```python
from build123d import *

# Parameters (mm, degrees)
SKETCH1_W           = 25
SKETCH1_H           = 68.1
BOSS_EXTRUDE1_DEPTH = 31.05
CUT_EXTRUDE1_REACH  = 54.426
SKETCH2_W           = 15
SKETCH2_H           = 26.05
SKETCH3_W           = 17
SKETCH3_H           = 21.05
CUT_EXTRUDE2_DEPTH  = 25
SKETCH7_W           = 25
SKETCH7_H           = 38.1
BOSS_EXTRUDE2_DEPTH = 5
SKETCH11_W          = 25
SKETCH11_H          = 15
CUT_EXTRUDE3_DEPTH  = 5
FILLET1_R           = 3.175
FILLET2_R           = 0.5
FILLET3_R           = 3.175


with BuildPart() as part:
    # Sketch1 → Boss-Extrude1 (new body)
    with BuildSketch(Plane(origin=(0, 0, 0), x_dir=(1, 0, 0), z_dir=(0, 1, 0))):
        Rectangle(SKETCH1_W, SKETCH1_H)
    extrude(amount=-BOSS_EXTRUDE1_DEPTH)

    # Sketch2 → Cut-Extrude1 (cut, up to next)
    with BuildSketch(Plane(origin=(12.5, 0, 0), x_dir=(0, 0, -1), z_dir=(1, 0, 0)), mode=Mode.PRIVATE) as cut_extrude1_sk1:
        with Locations((-26.55, -18.025)):
            Rectangle(SKETCH2_W, SKETCH2_H)
    cut_extrude1_tool1 = extrude(cut_extrude1_sk1.sketch, amount=-CUT_EXTRUDE1_REACH, mode=Mode.PRIVATE) & part.part
    # Sketch2 → Cut-Extrude1 (cut, up to next)
    with BuildSketch(Plane(origin=(12.5, 0, 0), x_dir=(0, 0, -1), z_dir=(1, 0, 0)), mode=Mode.PRIVATE) as cut_extrude1_sk2:
        with Locations((26.55, -18.025)):
            Rectangle(SKETCH2_W, SKETCH2_H)
    cut_extrude1_tool2 = extrude(cut_extrude1_sk2.sketch, amount=-CUT_EXTRUDE1_REACH, mode=Mode.PRIVATE) & part.part
    add(cut_extrude1_tool1.solids().sort_by_distance((12.5, -18.025, 26.55))[0], mode=Mode.SUBTRACT)
    add(cut_extrude1_tool2.solids().sort_by_distance((12.5, -18.025, -26.55))[0], mode=Mode.SUBTRACT)

    # Sketch3 → Cut-Extrude2 (cut, symmetric)
    with BuildSketch(Plane.XY):
        with Locations((-4, -15.525)):
            Rectangle(SKETCH3_W, SKETCH3_H)
    extrude(amount=CUT_EXTRUDE2_DEPTH, both=True, mode=Mode.SUBTRACT)

    # Sketch6 → Cut-Revolve2 (revolve, cut)
    with BuildSketch(Plane.XY, mode=Mode.PRIVATE) as cut_revolve2_sk:
        Polygon((-4, 0), (-4, -5), (-0.75, -5), (-0.75, -4), (1.5, -4), (1.5, 0), align=None)
    revolve(cut_revolve2_sk.sketch.rotate(Axis((-4, 0, 0), (0, -1, 0)), 180), axis=Axis((-4, 0, 0), (0, -1, 0)), mode=Mode.SUBTRACT)

    # Sketch7 → Boss-Extrude2 (add)
    with BuildSketch(Plane(origin=(0, 0, 0), x_dir=(1, 0, 0), z_dir=(0, 1, 0))):
        with Locations((25, 0)):
            Rectangle(SKETCH7_W, SKETCH7_H)
    extrude(amount=-BOSS_EXTRUDE2_DEPTH)

    # Sketch10 → Cut-Revolve3 (revolve, cut)
    with BuildSketch(Plane.XY, mode=Mode.PRIVATE) as cut_revolve3_sk:
        Polygon((25, 0), (19, 0), (22.75, -3.75), (22.75, -5), (25, -5), align=None)
    revolve(cut_revolve3_sk.sketch.rotate(Axis((25, -5, 0), (0, 1, 0)), 270), axis=Axis((25, -5, 0), (0, 1, 0)), mode=Mode.SUBTRACT)

    # Sketch11 → Cut-Extrude3 (cut)
    with BuildSketch(Plane(origin=(0, 0, 0), x_dir=(1, 0, 0), z_dir=(0, 1, 0))):
        with Locations((0, 26.55)):
            Rectangle(SKETCH11_W, SKETCH11_H)
        with Locations((0, -26.55)):
            Rectangle(SKETCH11_W, SKETCH11_H)
    extrude(amount=-CUT_EXTRUDE3_DEPTH, mode=Mode.SUBTRACT)

    # Fillet1
    fillet1_edges = [part.edges().sort_by_distance(p)[0] for p in [
        (12.5, -18.025, 19.05),
        (12.5, -18.025, -19.05),
    ]]
    fillet(fillet1_edges, radius=FILLET1_R)

    # Fillet2
    fillet2_edges = [part.edges().sort_by_distance(p)[0] for p in [
        (-4, -5, 19.05),
        (12.5, -31.05, 0),
        (11.57006403, -31.05, -18.12006403),
        (11.57006403, -31.05, 18.12006403),
        (-12.5, -31.05, 0),
        (-1.5875, -31.05, 19.05),
        (-1.5875, -31.05, -19.05),
        (-4, -26.05, 19.05),
        (-12.5, -26.05, 0),
        (-4, -26.05, -19.05),
        (12.5, 0, -19.05),
        (12.5, 0, 19.05),
        (37.5, 0, 0),
        (23.4125, -5, -19.05),
        (37.5, -5, 0),
        (23.4125, -5, 19.05),
        (-12.5, -5, 0),
        (-4, -5, -19.05),
        (-12.5, 0, 0),
    ]]
    fillet(fillet2_edges, radius=FILLET2_R)

    # Fillet3
    # the kernel refuses this fillet: 3.175 mm, written as the material it takes off along each edge
    with BuildSketch(Plane(origin=(-9.325, -31.05, -15.875), x_dir=(-1, 0, 0), z_dir=(0, 0, 1))) as fillet3_piece_1:
        with BuildLine():
            CenterArc((2.675, -0.5), 0.5, 0, 90)
            Line((3.175, -0.5), (3.175, 0))
            Line((3.175, 0), (2.675, 0))
        make_face()
    revolve(axis=Axis((-9.325, -31.05, -15.875), (0, -1, 0)), revolution_arc=90, mode=Mode.SUBTRACT)
    with BuildSketch(Plane(origin=(-9.325, -31.05, 15.875), x_dir=(0, 0, 1), z_dir=(1, 0, 0))) as fillet3_piece_2:
        with BuildLine():
            CenterArc((2.675, -0.5), 0.5, 0, 90)
            Line((3.175, -0.5), (3.175, 0))
            Line((3.175, 0), (2.675, 0))
        make_face()
    revolve(axis=Axis((-9.325, -31.05, 15.875), (0, -1, 0)), revolution_arc=90, mode=Mode.SUBTRACT)
    with BuildSketch(Plane(origin=(-9.325, -26.05, -15.875), x_dir=(0, 0, -1), z_dir=(1, 0, 0))) as fillet3_piece_3:
        with BuildLine():
            CenterArc((2.675, -0.5), 0.5, 0, 90)
            Line((3.175, -0.5), (3.175, 0))
            Line((3.175, 0), (2.675, 0))
        make_face()
    revolve(axis=Axis((-9.325, -26.05, -15.875), (0, 1, 0)), revolution_arc=90, mode=Mode.SUBTRACT)
    with BuildSketch(Plane(origin=(-9.325, -26.05, 15.875), x_dir=(-1, 0, 0), z_dir=(0, 0, -1))) as fillet3_piece_4:
        with BuildLine():
            CenterArc((2.675, -0.5), 0.5, 0, 90)
            Line((3.175, -0.5), (3.175, 0))
            Line((3.175, 0), (2.675, 0))
        make_face()
    revolve(axis=Axis((-9.325, -26.05, 15.875), (0, 1, 0)), revolution_arc=90, mode=Mode.SUBTRACT)
    with BuildSketch(Plane(origin=(-9.325, 0, 15.875), x_dir=(-1, 0, 0), z_dir=(0, 0, -1))) as fillet3_piece_5:
        with BuildLine():
            CenterArc((2.675, -0.5), 0.5, 0, 90)
            Line((3.175, -0.5), (3.175, 0))
            Line((3.175, 0), (2.675, 0))
        make_face()
    revolve(axis=Axis((-9.325, 0, 15.875), (0, 1, 0)), revolution_arc=90, mode=Mode.SUBTRACT)
    with BuildSketch(Plane(origin=(-9.325, 0, -15.875), x_dir=(0, 0, -1), z_dir=(1, 0, 0))) as fillet3_piece_6:
        with BuildLine():
            CenterArc((2.675, -0.5), 0.5, 0, 90)
            Line((3.175, -0.5), (3.175, 0))
            Line((3.175, 0), (2.675, 0))
        make_face()
    revolve(axis=Axis((-9.325, 0, -15.875), (0, 1, 0)), revolution_arc=90, mode=Mode.SUBTRACT)
    with BuildSketch(Plane(origin=(34.325, 0, 15.875), x_dir=(0, 0, 1), z_dir=(-1, 0, 0))) as fillet3_piece_7:
        with BuildLine():
            CenterArc((2.675, -0.5), 0.5, 0, 90)
            Line((3.175, -0.5), (3.175, 0))
            Line((3.175, 0), (2.675, 0))
        make_face()
    revolve(axis=Axis((34.325, 0, 15.875), (0, 1, 0)), revolution_arc=90, mode=Mode.SUBTRACT)
    with BuildSketch(Plane(origin=(34.325, 0, -15.875), x_dir=(1, 0, 0), z_dir=(0, 0, 1))) as fillet3_piece_8:
        with BuildLine():
            CenterArc((2.675, -0.5), 0.5, 0, 90)
            Line((3.175, -0.5), (3.175, 0))
            Line((3.175, 0), (2.675, 0))
        make_face()
    revolve(axis=Axis((34.325, 0, -15.875), (0, 1, 0)), revolution_arc=90, mode=Mode.SUBTRACT)
    with BuildSketch(Plane(origin=(-9.325, -5, 15.875), x_dir=(0, 0, 1), z_dir=(1, 0, 0))) as fillet3_piece_9:
        with BuildLine():
            CenterArc((2.675, -0.5), 0.5, 0, 90)
            Line((3.175, -0.5), (3.175, 0))
            Line((3.175, 0), (2.675, 0))
        make_face()
    revolve(axis=Axis((-9.325, -5, 15.875), (0, -1, 0)), revolution_arc=90, mode=Mode.SUBTRACT)
    with BuildSketch(Plane(origin=(-9.325, -5, -15.875), x_dir=(-1, 0, 0), z_dir=(0, 0, 1))) as fillet3_piece_10:
        with BuildLine():
            CenterArc((2.675, -0.5), 0.5, 0, 90)
            Line((3.175, -0.5), (3.175, 0))
            Line((3.175, 0), (2.675, 0))
        make_face()
    revolve(axis=Axis((-9.325, -5, -15.875), (0, -1, 0)), revolution_arc=90, mode=Mode.SUBTRACT)
    with BuildSketch(Plane(origin=(34.325, -5, -15.875), x_dir=(0, 0, -1), z_dir=(-1, 0, 0))) as fillet3_piece_11:
        with BuildLine():
            CenterArc((2.675, -0.5), 0.5, 0, 90)
            Line((3.175, -0.5), (3.175, 0))
            Line((3.175, 0), (2.675, 0))
        make_face()
    revolve(axis=Axis((34.325, -5, -15.875), (0, -1, 0)), revolution_arc=90, mode=Mode.SUBTRACT)
    with BuildSketch(Plane(origin=(34.325, -5, 15.875), x_dir=(1, 0, 0), z_dir=(0, 0, -1))) as fillet3_piece_12:
        with BuildLine():
            CenterArc((2.675, -0.5), 0.5, 0, 90)
            Line((3.175, -0.5), (3.175, 0))
            Line((3.175, 0), (2.675, 0))
        make_face()
    revolve(axis=Axis((34.325, -5, 15.875), (0, -1, 0)), revolution_arc=90, mode=Mode.SUBTRACT)
    with BuildSketch(Plane(origin=(37.5, 0, 19.05), x_dir=(0, 0, -1), z_dir=(0, -1, 0)), Plane(origin=(-12.5, -31.05, 19.05), x_dir=(0, 0, -1), z_dir=(0, 1, 0)), Plane(origin=(-12.5, -31.05, -19.05), x_dir=(1, 0, 0), z_dir=(0, 1, 0)), Plane(origin=(37.5, 0, -19.05), x_dir=(-1, 0, 0), z_dir=(0, -1, 0))) as fillet3_piece_13:
        with BuildLine():
            CenterArc((FILLET3_R, -FILLET3_R), FILLET3_R, 90, 90)
            Line((0, -FILLET3_R), (0, 0))
            Line((0, 0), (FILLET3_R, 0))
        make_face()
    extrude(amount=5, mode=Mode.SUBTRACT)
    with BuildSketch(Plane(origin=(-12.5, 0, 19.05), x_dir=(0, 0, -1), z_dir=(0, -1, 0)), Plane(origin=(-12.5, 0, -19.05), x_dir=(1, 0, 0), z_dir=(0, -1, 0))) as fillet3_piece_14:
        with BuildLine():
            CenterArc((FILLET3_R, FILLET3_R), FILLET3_R, 180, 90)
            Line((0, FILLET3_R), (0, 0))
            Line((0, 0), (FILLET3_R, 0))
        make_face()
    extrude(amount=5, mode=Mode.SUBTRACT)


solid = part.part
```
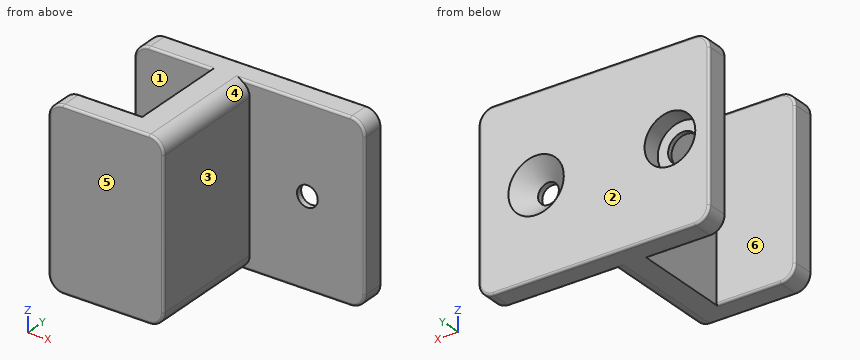
CAD build for the part. Positions are in the model's coordinates, mm. Face numbers are marked on the shaded views. A direction names the side the tool comes from. Round coordinates to 2 decimals unless told otherwise and drop trailing zeros. Order: outer loops, then holes, each group sorted by start corner. A loop starts at its lowest first (then second) coordinate and runs counter-clockwise, first axis right, second up.
Item 1: Saw through at B-B on z = 0. State how many separate pieces and enclosed holes the cut face has, then the cut area to 3 significant figures.
Item 2: Tool access for the marked faces 1, 2 and 3: list every direction of +Z, -Z, +X, -X, +Y, -Y with a clear straight run to the whole face (end or side of a thin tool).
Item 3: Saw through at C-C on x = -4. Write the cut outline in (y, z), then the cut area to 3 significant figures.
Item 4: Saw through at D-D on z = -14. Write the cut outline in (x, y).
Item 5: Saw through at A-A on x = 25. Write the cut outline in (y, z), then the cut area to 3 significant figures.
Item 6: Mould opens along Y. For the marked faces 4, 5 and 6 say: pulls with the +Y half, pulls with the -Y half, needs draft (parallel to the pull), parting line crosses it, or undercut.
Item 7: Probe line 1 along Y through (x, z) = (-3, -14); line 2 along X through (y, z) = (-1, -2); line 3 along Z through (x, y) = (-4, -4.6). List the from-to ranges inside material, lowest first.
Item 8: Pin check, flat tips, straight feed: pin 1 (8 mm diameter, centred on x = 23, z = 0, fed in from -Y); pin 2 (9 mm diameter, centred on x = -2, z = -1.5, fed in from +Y); pin 3 (1 mm diameter, centred on x = 12, y = -7, fed in from +Z); pin 4 (10.5 mm diameter, centred on x = -4, z = 0, fed in from +Y). Stop position of each tip, or through.
Reported:
1. separate pieces: 3
1. enclosed holes: 0
1. area: 456 mm2
2. face 1: +Z, -Z, -X
2. face 2: +Z, -Z, +X, -X, +Y
2. face 3: +Z, -Z, +X, -Y
3. outline: (-31.05, -18.55) arc R0.5 ccw to (-30.55, -19.05) - (-26.55, -19.05) arc R0.5 ccw to (-26.05, -18.55) - (-26.05, 18.55) arc R0.5 ccw to (-26.55, 19.05) - (-30.55, 19.05) arc R0.5 ccw to (-31.05, 18.55) - close; (-5, -18.55) arc R0.5 ccw to (-4.5, -19.05) - (-0.5, -19.05) arc R0.5 ccw to (0, -18.55) - (0, -5.5) - (-4, -5.5) - (-4, -3.25) - (-5, -3.25) - close; (-5, 3.25) - (-4, 3.25) - (-4, 5.5) - (0, 5.5) - (0, 18.55) arc R0.5 ccw to (-0.5, 19.05) - (-4.5, 19.05) arc R0.5 ccw to (-5, 18.55) - close
3. area: 330 mm2
4. outline: (-12.5, -30.55) arc R0.5 ccw to (-12, -31.05) - (12, -31.05) arc R0.5 ccw to (12.5, -30.55) - (12.5, -5) - (37, -5) arc R0.5 ccw to (37.5, -4.5) - (37.5, -0.5) arc R0.5 ccw to (37, 0) - (-12, 0) arc R0.5 ccw to (-12.5, -0.5) - (-12.5, -4.5) arc R0.5 ccw to (-12, -5) - (4.5, -5) - (4.5, -26.05) - (-12, -26.05) arc R0.5 ccw to (-12.5, -26.55) - close
5. outline: (-5, -18.55) arc R0.5 ccw to (-4.5, -19.05) - (-0.5, -19.05) arc R0.5 ccw to (0, -18.55) - (0, -6) - (-3.75, -2.25) - (-5, -2.25) - close; (-5, 2.25) - (-3.75, 2.25) - (0, 6) - (0, 18.55) arc R0.5 ccw to (-0.5, 19.05) - (-4.5, 19.05) arc R0.5 ccw to (-5, 18.55) - close
5. area: 154 mm2
6. face 4: needs draft
6. face 5: pulls with the -Y half
6. face 6: undercut
7. line 1: y = -31.05 to -26.05, -5 to 0
7. line 2: x = -12.5 to -9.12, 1.12 to 20.42, 29.58 to 37.5
7. line 3: z = -19.04 to -3.25, 3.25 to 19.04
8. pin 1: stops at y = -5
8. pin 2: stops at y = 0
8. pin 3: stops at z = 18.19
8. pin 4: stops at y = -4
